The model under review builds one solid part; all positions refer to its coordinate system, in mm. Face numbers are marked on the shaded views. A direction names the side the tool comes from. Give positions to 0.01 mm unless a question says otherwise; leave off trailing zeros. Loops run counter-clockwise (first coordinate to the right, second up) from the corner with the lowest first, then second, coordinate; pieces in that order, holes last. Notation, with made-up numbers: M -13,59 L -8,59 A12 cw -8,76 Z; hole C 82.5,-6 d3. An arc over 180 degrees is marked long. One line per item, written item: value. Start each with the question number.
Q1. For pin 1 (4.5 mm diameter, centred on x = 120, y = 144, fed in from +Z); pin 2 (0.8 mm diameter, centred on x = 89, z = 28.5, fed in from -Y); pin 3 (1.5 mm diameter, centred on x = 114.5, y = 21.5, fed in from -Z); pin 4 (2.5 mm diameter, centred on x = 40, y = 119, fed in from +Z), all flat-tipped, find the tip position at first contact; note any pin that passes through.
Q2. We need section C-C on y = 129.5. Write out the cut boundary in (x, z), plus the area to 3 significant figures.
Q3. We need section D-D on y = 86.5. Write out the cut boundary in (x, z), plus the area to 3 significant figures.
Q4. For the marked faces 4 and 5, list the 3-axis set-ups (+Z, -Z, +X, -X, +Y, -Y) from which the entire face can be reached by the end or side of a thin tool; tool diameter is ignored.
Q5. To check wall thickness, follow line 1 along X through (y, z) = (144, 27.45); line 2 along X through (y, z) = (21.5, 20.5). State the ranges of each line that lie inside material, in increasing order. Write a range as from..to.
Q6. Mouldability with a two-part tool opening along Y and no side actions: class the marked faces 1, 2 and 3 as released by +Y, released by -Y, zero draft, split by the parting line, or undercut.
Q7. We need section B-B on z = 5. Write out the cut boundary in (x, y).
Q8. We need section A-A on x = 94.5. Write out the cut boundary in (y, z).
Autodesk Fusion 360 part; units mm, degrees
sketch "Sketch1" plane through (0, 0, 0) normal (0, 0, 1) x (1, 0, 0)
  line L0 (0, 0) -> (160, 0)
  line L1 (160, 0) -> (160, 160)
  line L2 (160, 160) -> (0, 160)
  line L3 (0, 160) -> (0, 0)
  dimension "d1" = 160
  dimension "d3" = 160
extrude "Extrude1" add sketch "Sketch1" along normal blind 30
fillet "Fillet1" radius 5 4 edges at (0, 160, 15) (0, 0, 15) (160, 0, 15) (160, 160, 15)
fillet "Fillet1" radius 3 4 edges at (160, 80, 30) (80, 160, 30) (80, 0, 30) (0, 80, 30)
shell "Shell1" thickness 2.7 removed faces 1 at (53.3333, 51.6667, 0)
sketch "Sketch3" plane through (0, 0, 30) normal (0, 0, 1) x (-1, 0, 0)
  arc A0 (-5, -157) -> (-3, -155) centre (-5, -155) ccw
  line L0 (-3, -155) -> (-3, -5)
  arc A1 (-3, -5) -> (-5, -3) centre (-5, -5) ccw
  line L1 (-5, -3) -> (-155, -3)
  arc A2 (-155, -3) -> (-157, -5) centre (-155, -5) ccw
  line L2 (-157, -5) -> (-157, -155)
  arc A3 (-157, -155) -> (-155, -157) centre (-155, -155) ccw
  line L3 (-155, -157) -> (-5, -157)
  line L4 (-44, -145) -> (-116, -145)
  line L5 (-116, -145) -> (-116, -118)
  line L6 (-116, -118) -> (-44, -118)
  line L7 (-44, -118) -> (-44, -145)
  arc A4 (-155, 0) -> (-160, -5) centre (-155, -5) ccw
  line L8 (-160, -5) -> (-160, -155)
  arc A5 (-160, -155) -> (-155, -160) centre (-155, -155) ccw
  line L9 (-155, -160) -> (-5, -160)
  arc A6 (-5, -160) -> (0, -155) centre (-5, -155) ccw
  line L10 (0, -155) -> (0, -5)
  arc A7 (0, -5) -> (-5, 0) centre (-5, -5) ccw
  line L11 (-5, 0) -> (-155, 0)
  line L12 (-80, -145) -> (-80, -160) construction
  dimension "d11" = 72
  dimension "d12" = 27
  dimension "d13" = 15
extrude "Extrude2" cut sketch "Sketch3" along normal through all and the other way through all contours L4 L5 L6 L7
sketch "Sketch4" plane through (0, 0, 30) normal (0, 0, 1) x (-1, 0, 0)
  line L0 (-44, -145) -> (-44, -118)
  line L1 (-44, -118) -> (-116, -118)
  line L2 (-116, -118) -> (-116, -145)
  line L3 (-116, -145) -> (-44, -145)
  arc A0 (-155, 0) -> (-160, -5) centre (-155, -5) ccw
  line L4 (-160, -5) -> (-160, -155)
  arc A1 (-160, -155) -> (-155, -160) centre (-155, -155) ccw
  line L5 (-155, -160) -> (-5, -160)
  arc A2 (-5, -160) -> (0, -155) centre (-5, -155) ccw
  line L6 (0, -155) -> (0, -5)
  arc A3 (0, -5) -> (-5, 0) centre (-5, -5) ccw
  line L7 (-5, 0) -> (-155, 0)
  line L8 (-40, -144) -> (-120, -144)
  line L9 (-120, -144) -> (-120, -119)
  line L10 (-120, -119) -> (-40, -119)
  line L11 (-40, -119) -> (-40, -144)
  line L12 (-44, -131.5) -> (-40, -131.5)
  line L13 (-80, -144) -> (-80, -145)
  line L14 (-80, -118) -> (-80, -119)
  line L15 (-116, -131.5) -> (-120, -131.5)
  dimension "d31" = 80
  dimension "d32" = 25
sketch "Sketch5" plane through (0, 0, 30) normal (0, 0, 1) x (-1, 0, 0)
  line L0 (-44, -118) -> (-44, -145)
  line L1 (-44, -145) -> (-116, -145)
  line L2 (-116, -145) -> (-116, -118)
  line L3 (-116, -118) -> (-44, -118)
  arc A0 (-5, -157) -> (-3, -155) centre (-5, -155) ccw
  line L4 (-3, -155) -> (-3, -5)
  arc A1 (-3, -5) -> (-5, -3) centre (-5, -5) ccw
  line L5 (-5, -3) -> (-155, -3)
  arc A2 (-155, -3) -> (-157, -5) centre (-155, -5) ccw
  line L6 (-157, -5) -> (-157, -155)
  arc A3 (-157, -155) -> (-155, -157) centre (-155, -155) ccw
  line L7 (-155, -157) -> (-5, -157)
  circle A4 centre (-45.1225, -143.8775) radius 1.5875
  line L8 (-44, -145) -> (-45.1225, -143.8775)
  circle A5 centre (-114.8775, -143.8775) radius 1.5875
  line L9 (-116, -145) -> (-114.8775, -143.8775) construction
  dimension "d23" = 3.175
  dimension "d24" = 45
  dimension "d25" = 3.175
extrude "Extrude3" cut sketch "Sketch5" along normal through all and the other way through all contours L0 A4 | L0 L1 A4 | L1 A4 | L1 L2 A5 | L2 A5 | L1 A5
ref_plane "WorkPlane1" through (80, 131.5, 28.65) normal (0, -1, 0) x (-1, 0, 0)
mirror "Mirror1" about plane through (80, 131.5, 28.65) normal (0, -1, 0) of "Extrude3"
fillet "Fillet2" [suppressed]
hole "Hole1" at (120, 144, 30) at (120, 119, 30) at (40, 119, 30) at (40, 144, 30) direction (0, 0, -1) diameter 3.4 depth 15 tip angle 118 countersink diameter 7.5 countersink angle 90
equation "d1 = Lid_X"
equation "d3 = Lid_Y"
equation "d4 = Lid_Z"
equation "d8 = Lid_Thikness"
equation "d11 = Opening_X"
equation "d12 = Opening_Y"
equation "d23 = d25"
equation "d25 = dog_bone_DIA"
equation "d30 = Corner_rad"
equation "d31 = Holes_X"
equation "d32 = Holes_Y"
equation "Lid_X = 160 mm"
equation "Lid_Y = 160 mm"
equation "Lid_Z = 30 mm"
equation "Opening_X = 72 mm"
equation "Opening_Y = 27 mm"
equation "Lid_Thikness = 2.7 mm"
equation "Corner_rad = 0.793 mm"
equation "Holes_X = 80 mm"
equation "Holes_Y = 25 mm"
equation "dog_bone_DIA = 0'- 1/8\""
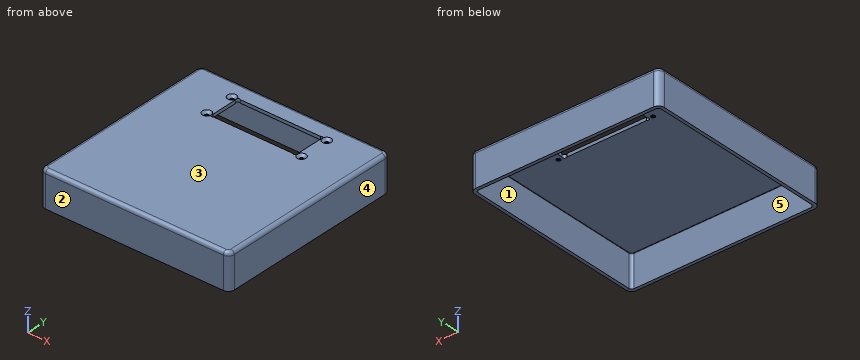
Solved:
1. pin 1: z = 28.5
1. pin 2: y = 0.21
1. pin 3: z = 27.3
1. pin 4: through
2. outline: M 0,0 L 2.7,0 L 2.7,27 A0.3 cw 3,27.3 L 44,27.3 L 44,30 L 3,30 A3 ccw 0,27 Z; M 116,27.3 L 157,27.3 A0.3 cw 157.3,27 L 157.3,0 L 160,0 L 160,27 A3 ccw 157,30 L 116,30 Z
2. area: 381 mm2
3. outline: M 0,0 L 2.7,0 L 2.7,27 A0.3 cw 3,27.3 L 157,27.3 A0.3 cw 157.3,27 L 157.3,0 L 160,0 L 160,27 A3 ccw 157,30 L 3,30 A3 ccw 0,27 Z
3. area: 576 mm2
4. face 4: +Z, -Z, +X, +Y, -Y
4. face 5: -Z
5. line 1: 0.03..38.3, 41.7..43.54, 116.46..118.3, 121.7..159.97
5. line 2: 0..2.7, 157.3..160
6. face 1: undercut
6. face 2: released by -Y
6. face 3: zero draft
7. outline: M 0,5 A5 ccw 5,0 L 155,0 A5 ccw 160,5 L 160,155 A5 ccw 155,160 L 5,160 A5 ccw 0,155 Z; hole M 2.7,5 A2.3 ccw 5,2.7 L 155,2.7 A2.3 ccw 157.3,5 L 157.3,155 A2.3 ccw 155,157.3 L 5,157.3 A2.3 ccw 2.7,155 Z
8. outline: M 0,0 L 2.7,0 L 2.7,27 A0.3 cw 3,27.3 L 118,27.3 L 118,30 L 3,30 A3 ccw 0,27 Z; M 145,27.3 L 157,27.3 A0.3 cw 157.3,27 L 157.3,0 L 160,0 L 160,27 A3 ccw 157,30 L 145,30 Z
